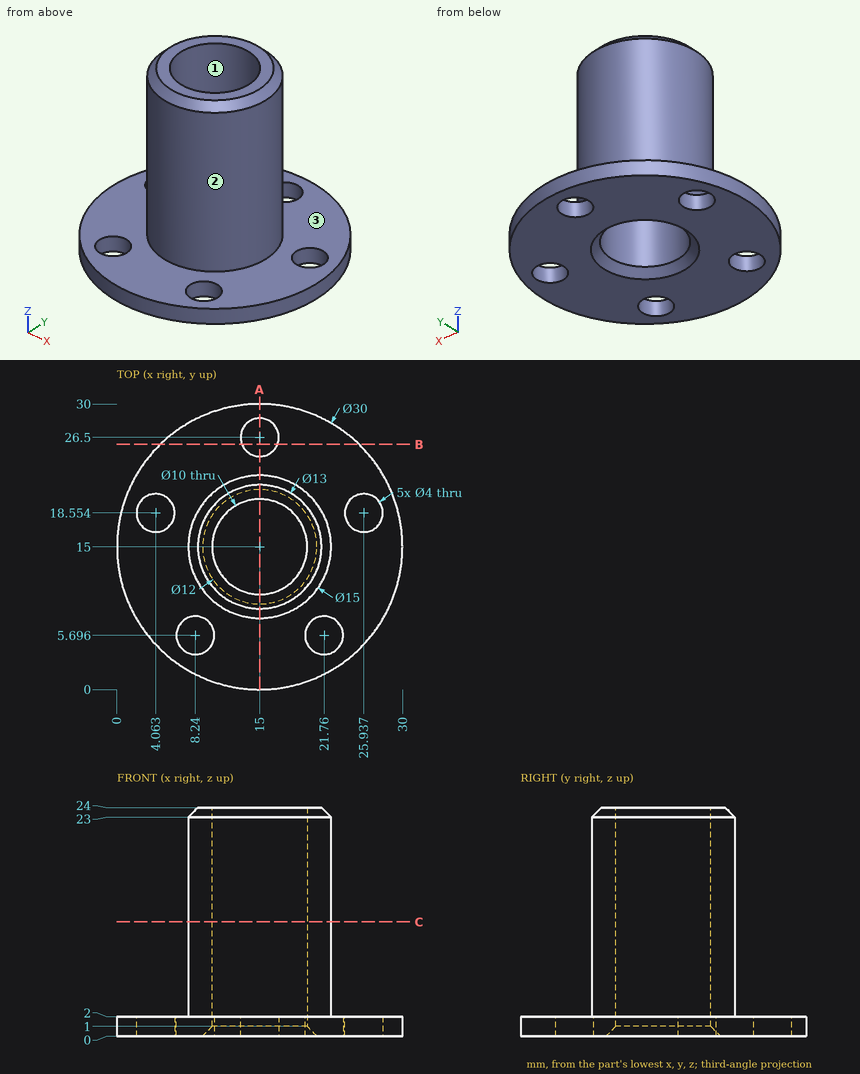
Geometry check sheet. Reference: drawing and pictorial views, mm from the part's lowest x, y, z. Give positions to 0.01 mm unless a question says otherwise; leave off trailing zeros. Loops run counter-clockwise (first coordinate to the right, second up) from the corner with the lowest first, then second, coordinate; pieces in that order, holes last.
1. Section check B-B, the plane y = 25.75. Enter the section's corners in (x, z).
2. Mould release check, pull along Y, two halves, no side actions. Record for the marked faces 1, 2 and 3: released by +Y, released by -Y, zero draft, split by the parting line, or undercut.
3. Section check C-C, the plane z = 12. Enter the section's corners in (x, y).
4. Thickness scan on line 1 (Y direction, x = 15.25, z = 22.5) (1 decimal); line 2 (Y direction, x = 15, z = 0.6); line 3 (Y direction, x = 15, z = 0.85). Record the ranges inside material, lowest first.
5. Section check A-A, the plane x = 15. Enter the section's corners in (y, z), then the cut area to 3 significant figures.
6. Go/stop test with flat-tipped pins: pin 1 Ø1.5 at (x, y) = (15.5, 4) entering from +Z; pin 2 Ø12 at (x, y) = (17, 23.5) entering from +Z; pin 3 Ø12 at (x, z) = (18.5, 10) entering from -Y; pin 4 Ø6 at (y, z) = (9, 12.5) entering from +X. Record where each tip stops, or that it passes through.
Geometry says:
1. outline: (4.54, 0) - (13.15, 0) - (13.15, 2) - (4.54, 2) - close; (16.85, 0) - (25.46, 0) - (25.46, 2) - (16.85, 2) - close
2. face 1: undercut
2. face 2: split by the parting line
2. face 3: zero draft
3. outline: circle Ø15 at (15, 15); hole circle Ø10 at (15, 15)
4. line 1: y = 7.5 to 10, 20 to 22.5
4. line 2: y = 0 to 9.6, 20.4 to 24.5, 28.5 to 30
4. line 3: y = 0 to 9.85, 20.15 to 24.5, 28.5 to 30
5. outline: (0, 0) - (9, 0) - (10, 1) - (10, 24) - (8.5, 24) - (7.5, 23) - (7.5, 2) - (0, 2) - close; (20, 1) - (21, 0) - (24.5, 0) - (24.5, 2) - (22.5, 2) - (22.5, 23) - (21.5, 24) - (20, 24) - close; (28.5, 0) - (30, 0) - (30, 2) - (28.5, 2) - close
5. area: 140 mm2
6. pin 1: stops at z = 2
6. pin 2: stops at z = 24
6. pin 3: stops at y = 7.5
6. pin 4: stops at x = 21.87
